from build123d import *

# Parameters (mm, degrees)
SKETCH_1_R               = 18
SKETCH_1_R_2             = 1.6
EXTRUDE_1_DEPTH          = 3
HOLE_WIZARD_2_AT_2_COUNT = 2
HOLE_WIZARD_2_AT_2_PITCH = 24.248711306
HOLE_WIZARD_2_AT_3_COUNT = 2
HOLE_WIZARD_2_AT_3_PITCH = 24.248711306
SKETCH_9_R               = 5.1
EXTRUDE_2_DEPTH          = 6


with BuildPart() as part:
    # 草图1 → 凸台-拉伸1 (new body)
    with BuildSketch(Plane(origin=(0, 0, 0), x_dir=(1, 0, 0), z_dir=(0, 1, 0))):
        with Locations(Location((0, 0, 0), (0, 0, 270))):
            Circle(SKETCH_1_R)
        with BuildLine():
            Line((-1.532970972, 2.1), (1.532970972, 2.1))
            ThreePointArc((1.532970972, 2.1), (0, -2.6), (-1.532970972, 2.1))
        make_face(mode=Mode.SUBTRACT)
        with Locations(Location((-12.124355653, -7, 0), (0, 0, 270))):
            Circle(SKETCH_1_R_2, mode=Mode.SUBTRACT)
        with Locations(Location((12.124355653, -7, 0), (0, 0, 270))):
            Circle(SKETCH_1_R_2, mode=Mode.SUBTRACT)
        with Locations(Location((0, 14, 0), (0, 0, 270))):
            Circle(SKETCH_1_R_2, mode=Mode.SUBTRACT)
    extrude(amount=EXTRUDE_1_DEPTH)

    # 草图8 → 打孔尺寸(%根据十字)槽沉头木螺钉的类型2 (revolve, cut)
    with BuildSketch(Plane(origin=(12.124355653, 0, 7), x_dir=(0, 0, -1), z_dir=(1, 0, 0))):
        Polygon((0, 0), (0, 3), (1.7, 3), (1.7, 1.6), (3.3, 0), align=None)
    hole_wizard_2 = revolve(axis=Axis((12.124355653, -6.35, 7), (0, 1, 0)), mode=Mode.SUBTRACT)

    # 打孔尺寸(%根据十字)槽沉头木螺钉的类型2 at 2: 打孔尺寸(%根据十字)槽沉头木螺钉的类型2 ×2
    with Locations(*[(-i * HOLE_WIZARD_2_AT_2_PITCH, 0, 0) for i in range(1, HOLE_WIZARD_2_AT_2_COUNT)]):
        add(hole_wizard_2, mode=Mode.SUBTRACT)

    # 打孔尺寸(%根据十字)槽沉头木螺钉的类型2 at 3: 打孔尺寸(%根据十字)槽沉头木螺钉的类型2 ×2
    with Locations(*[Vector(-0.5000000000000048, 0, -0.8660254037844359) * (i * HOLE_WIZARD_2_AT_3_PITCH) for i in range(1, HOLE_WIZARD_2_AT_3_COUNT)]):
        add(hole_wizard_2, mode=Mode.SUBTRACT)

    # 草图9 → 凸台-拉伸2 (add)
    with BuildSketch(Plane(origin=(0, 3, 0), x_dir=(1, 0, 0), z_dir=(0, 1, 0))):
        with Locations(Location((0, 0, 0), (0, 0, 270))):
            Circle(SKETCH_9_R)
        with BuildLine():
            Line((-1.532970972, 2.1), (1.532970972, 2.1))
            ThreePointArc((1.532970972, 2.1), (0, -2.6), (-1.532970972, 2.1))
        make_face(mode=Mode.SUBTRACT)
    extrude(amount=EXTRUDE_2_DEPTH)


solid = part.part
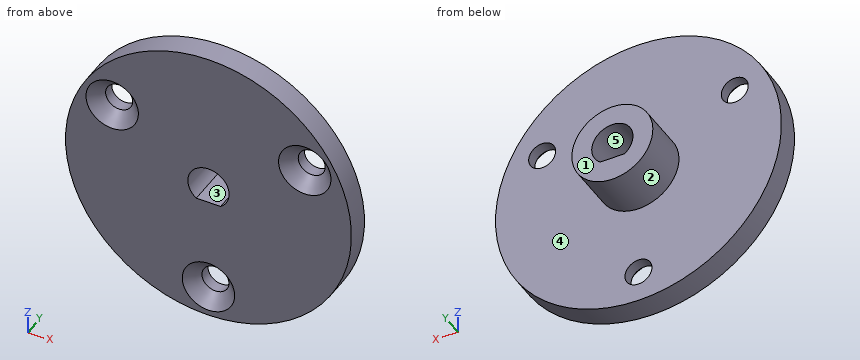
Read the model definition and answer for the solid it produces. Units are mm, in the model's axes. Face numbers are marked on the shaded views. A direction names the side the tool comes from. Round coordinates to 2 decimals unless told otherwise and drop trailing zeros. Write each loop counter-clockwise with the first axis right and the second up, starting at its lowest first coordinate (ties: lowest second). Pieces come first, ordered by that corner, then holes. Notation, with made-up numbers: (76, 42.25) - (85, 42.25) arc R13 ccw to (85, 61.25) - close; hole circle Ø4 at (-10.5, 39). An arc over 180 degrees is marked (long way). Use a Markdown table: item, result.
(1) The mould has two halves that part along X. Classify the marked faces 1, 2 and 3: released by +X, released by -X, zero draft, split by the parting line, or undercut.
Reported:
| item | result |
|---|---|
| face 1 | zero draft |
| face 2 | split by the parting line |
| face 3 | undercut |
(2) The part is cut by section B-B (x = 0). Write down the section's boundary in (y, z).
Reported:
| item | result |
|---|---|
| outline | (0, -18) - (3, -18) - (3, -15.7) - (1.6, -15.7) - (0, -17.3) - close; (0, -10.7) - (1.6, -12.3) - (3, -12.3) - (3, -5.1) - (9, -5.1) - (9, -2.1) - (0, -2.1) - close; (0, 2.6) - (9, 2.6) - (9, 5.1) - (3, 5.1) - (3, 18) - (0, 18) - close |
(3) Straight lines are drawn through the part: line 1 along Z through (x, y) = (0.5, 1.25); line 2 along X through (y, z) = (1.95, -14); line 3 along Z through (x, y) = (-1, 3.25). For each, find the intervals that lie inside material, in ascending order. Write a range as [from, to].
Reported:
| item | result |
|---|---|
| line 1 | [-17.99, -15.99], [-12.01, -2.1], [2.55, 17.99] |
| line 2 | [-11.31, -1.7], [1.7, 11.31] |
| line 3 | [-5, -2.1], [2.4, 5] |
(4) The part is cut by section D-D (z = 7). Write down the section's boundary in (x, y), then the cut area to 3 significant figures.
Reported:
| item | result |
|---|---|
| outline | (-16.58, 0) - (-15.42, 0) - (-13.82, 1.6) - (-13.82, 3) - (-16.58, 3) - close; (-10.42, 1.6) - (-8.82, 0) - (8.82, 0) - (10.42, 1.6) - (10.42, 3) - (-10.42, 3) - close; (13.82, 1.6) - (15.42, 0) - (16.58, 0) - (16.58, 3) - (13.82, 3) - close |
| area | 74.0 mm2 |
(5) Each of these flat-tipped pins is pushed along its axis until it touches: pin 1 Ø3 at (x, z) = (-12.12, 7) entering from -Y; pin 2 Ø4 at (x, z) = (12.12, 7) entering from -Y; pin 3 Ø3 at (y, z) = (1, 5) entering from +X; pin 4 Ø2 at (y, z) = (1, -4.5) entering from -X. Where does it stop, or does it pass through?
Reported:
| item | result |
|---|---|
| pin 1 | through |
| pin 2 | y = 1.3 |
| pin 3 | x = 17.66 |
| pin 4 | x = -17.66 |
(6) The part is cut by section A-A (z = 0). Write down the section's boundary in (x, y), then the cut area to 3 significant figures.
Reported:
| item | result |
|---|---|
| outline | (-18, 0) - (-2.6, 0) - (-2.6, 9) - (-5.1, 9) - (-5.1, 3) - (-18, 3) - close; (2.6, 0) - (18, 0) - (18, 3) - (5.1, 3) - (5.1, 9) - (2.6, 9) - close |
| area | 122 mm2 |
(7) Which of the six approach directions +Z, -Z, +X, -X, +Y, -Y give full straight-line access (tool end or side, diameter ignored) to the marked faces 4 and 5?
Reported:
| item | result |
|---|---|
| face 4 | +Y |
| face 5 | +Y, -Y |
(8) The part is cut by section C-C (y = 5). Write down the section's boundary in (x, z).
Reported:
| item | result |
|---|---|
| outline | circle Ø10.2 at (0, 0); hole (-1.53, -2.1) - (1.53, -2.1) arc R2.6 ccw (long way) to start |
